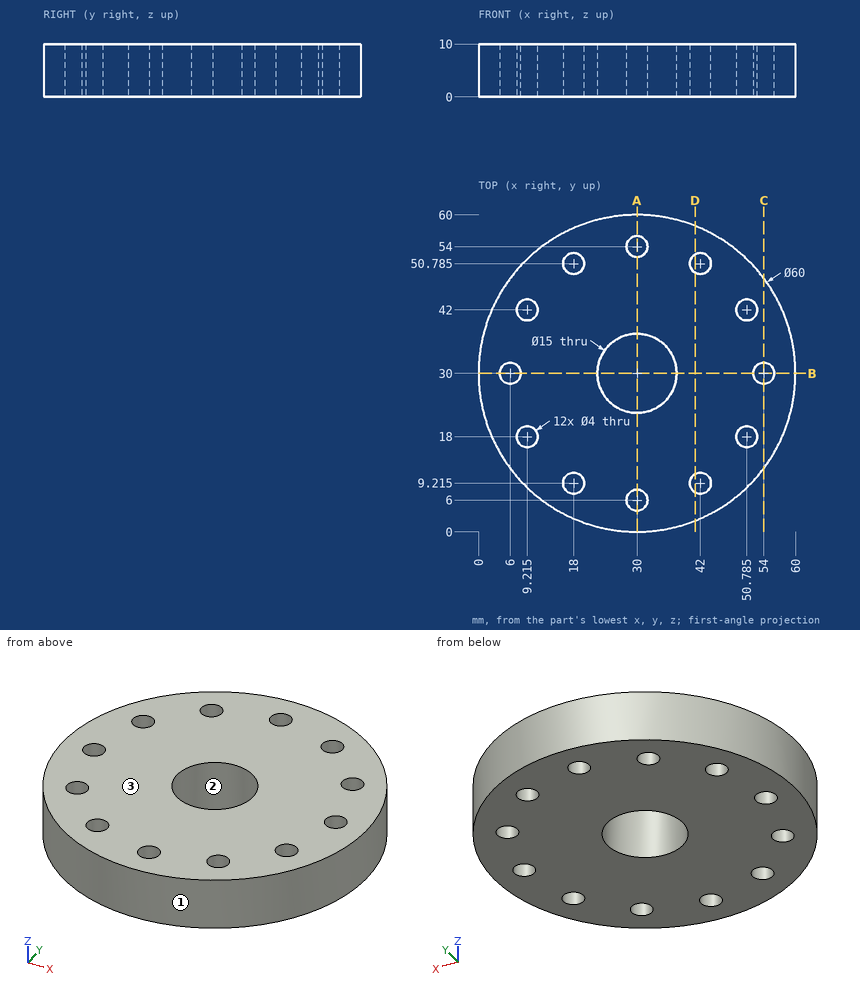
Geometry: see drawing. Coordinates: mm, zero at the bounding-box minimum. Give positions to 0.01 mm unless a question says otherwise; leave off trailing zeros. Write each loop counter-clockwise with the first axis right and the second up, starting at its lowest first coordinate (ties: lowest second). Pieces come first, ordered by that corner, then holes. Notation, with made-up numbers: (15.25, 43.25) - (40.25, 43.25) arc R26 ccw to (40.25, 76.25) - close; hole circle Ø2 at (-21, 85.5). An arc over 180 degrees is marked (long way). Return JSON: item names as keys, results as strings. Group by question number.
1) Section D-D on x = 41. Return the cut outline in (y, z), plus the area to 3 significant figures.
2) Mould query, pull axis Y, two halves, no side actions, for the marked faces 1, 2 and 3. Classes: released by +Y, released by -Y, zero draft, split by the parting line, or undercut.
3) Section A-A on x = 30. Return the cut outline in (y, z), plus the area to 3 significant figures.
4) Section C-C on x = 54. Return the cut outline in (y, z).
5) First-contact query: P1, Ø6, axis at x = 51, z = 7.5, coming from the +Y side; P2, Ø4, axis at x = 29, z = 6.5, coming from the -Y side; P3, Ø3.5, axis at x = 42, y = 9.22, coming from the +Z side; P4, Ø6, axis at x = 19, z = 1, coming from the -Y side. Flat tips, straight axial feed; report the tip coordinate or a pass-through.
6) Line query: line 1 (Y direction, x = 30, z = 7); line 2 (X direction, y = 29, z = 4.5) (1 decimal); line 3 (X direction, y = 42, z = 7.75) (1 decimal). Output: solid intervals per line, ascending.
Filled in:
{
 "1": {"outline": "(2.09, 0) - (7.48, 0) - (7.48, 10) - (2.09, 10) - close; (10.95, 0) - (49.05, 0) - (49.05, 10) - (10.95, 10) - close; (52.52, 0) - (57.91, 0) - (57.91, 10) - (52.52, 10) - close", "area": "489 mm^2"},
 "2": {"face 1": "split by the parting line", "face 2": "undercut", "face 3": "zero draft"},
 "3": {"outline": "(0, 0) - (4, 0) - (4, 10) - (0, 10) - close; (8, 0) - (22.5, 0) - (22.5, 10) - (8, 10) - close; (37.5, 0) - (52, 0) - (52, 10) - (37.5, 10) - close; (56, 0) - (60, 0) - (60, 10) - (56, 10) - close", "area": "370 mm^2"},
 "4": {"outline": "(12, 0) - (28, 0) - (28, 10) - (12, 10) - close; (32, 0) - (48, 0) - (48, 10) - (32, 10) - close"},
 "5": {"P1": "stops at y = 54", "P2": "stops at y = 0", "P3": "passes through", "P4": "stops at y = 1.09"},
 "6": {"line 1": "y = 0 to 4, 8 to 22.5, 37.5 to 52, 56 to 60", "line 2": "x = 0 to 4.3, 7.7 to 22.6, 37.4 to 52.3, 55.7 to 60", "line 3": "x = 2.5 to 7.2, 11.2 to 48.8, 52.8 to 57.5"}
}
